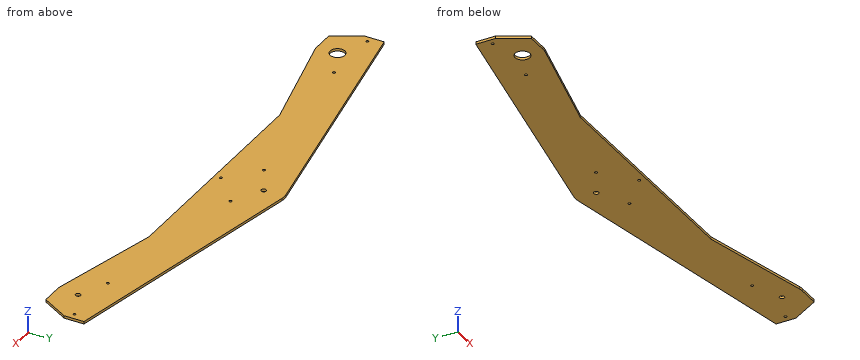
from build123d import *

# Parameters (mm, degrees)
MODEL_R             = 14.2875
MODEL_R_2           = 4.7625
MODEL_R_3           = 2.5527
BOSS_EXTRUDE1_DEPTH = 4.7752


with BuildPart() as part:
    # Model → Boss-Extrude1 (new body)
    with BuildSketch(Plane.XY):
        with BuildLine():
            Line((379.149829152, 1141.15149464), (590.378339475, 1192.375592492))
            Line((590.378339475, 1192.375592492), (814.376062419, 1192.375592492))
            Line((814.376062419, 1192.375592492), (1038.373785363, 1192.375592492))
            Line((1038.373785363, 1192.375592492), (1249.602295686, 1141.15149464))
            ThreePointArc((1249.602295686, 1141.15149464), (1254.256081724, 1140.312171612), (1258.976587117, 1140.031072925))
            Line((1258.976587117, 1140.031072925), (1298.696307446, 1140.031072925))
            Line((1298.696307446, 1140.031072925), (1328.726062419, 1192.375592492))
            Line((1328.726062419, 1192.375592492), (1328.726062419, 1230.475592492))
            Line((1328.726062419, 1230.475592492), (821.794166075, 1326.704151001))
            ThreePointArc((821.794166075, 1326.704151001), (814.376062419, 1327.401992492), (806.957958762, 1326.704151001))
            Line((806.957958762, 1326.704151001), (300.026062419, 1230.475592492))
            Line((300.026062419, 1230.475592492), (300.026062419, 1192.375592492))
            Line((300.026062419, 1192.375592492), (330.055817392, 1140.031072925))
            Line((330.055817392, 1140.031072925), (369.775537721, 1140.031072925))
            ThreePointArc((369.775537721, 1140.031072925), (374.496043114, 1140.312171612), (379.149829152, 1141.15149464))
        make_face()
        with Locations((369.877137721, 1179.807472925)):
            Circle(MODEL_R, mode=Mode.SUBTRACT)
        with Locations((814.376062419, 1287.625592492)):
            Circle(MODEL_R_2, mode=Mode.SUBTRACT)
        with Locations((1258.874987117, 1179.807472925)):
            Circle(MODEL_R_2, mode=Mode.SUBTRACT)
        with Locations((1201.72498751, 1205.075592492)):
            Circle(MODEL_R_3, mode=Mode.SUBTRACT)
        with Locations((1316.024986723, 1205.075592492)):
            Circle(MODEL_R_3, mode=Mode.SUBTRACT)
        with Locations((757.227138115, 1255.875592492)):
            Circle(MODEL_R_3, mode=Mode.SUBTRACT)
        with Locations((871.524986723, 1255.875592492)):
            Circle(MODEL_R_3, mode=Mode.SUBTRACT)
        with Locations((814.376062419, 1205.075592492)):
            Circle(MODEL_R_3, mode=Mode.SUBTRACT)
        with Locations((312.727138115, 1205.075592492)):
            Circle(MODEL_R_3, mode=Mode.SUBTRACT)
        with Locations((427.027137328, 1205.075592492)):
            Circle(MODEL_R_3, mode=Mode.SUBTRACT)
    extrude(amount=BOSS_EXTRUDE1_DEPTH)


solid = part.part
Design review of the part built by this model. Coordinates are the model's own, in mm. Give positions to 0.01 mm unless a question says otherwise; leave off trailing zeros. Loops run counter-clockwise (first coordinate to the right, second up) from the corner with the lowest first, then second, coordinate; pieces in that order, holes last. Notation, with made-up numbers: M -30.5,-38 L -4.5,-38 A10 ccw -4.5,-29 Z; hole C -18,52.25 d2. An arc over 180 degrees is marked long. Answer as a JSON object with one key per item and string values.
Item 1: We need section A-A (z = 3.8). Count the separate pieces of the cut face and the enclosed holes in it, and give its area (3 significant figures).
Output values:
{"separate pieces": "1", "enclosed holes": "10", "area": "106,000 mm2"}
Item 2: For P1, Ø6, axis at x = 603.5, y = 1260.5, coming from the -Z side; P2, Ø3, axis at x = 757.23, y = 1255.88, coming from the -Z side, all flat-tipped, find the tip position at first contact; note any pin that passes through.
Output values:
{"P1": "stops at z = 0", "P2": "passes through"}
Item 3: We need section B-B (x = 657). State the section outline as (y, z) points, and give its area (3 significant figures).
Output values:
{"outline": "M 1192.38,0 L 1298.24,0 L 1298.24,4.78 L 1192.38,4.78 Z", "area": "506 mm2"}
Item 4: Wall thickness on line 1 along X through (y, z) = (1203.5, 3.25); line 2 along Y through (x, z) = (1234, 1.35); line 3 along Y through (x, z) = (808, 1.65): over which ranges is each line inside the solid? List them lowest first.
Output values:
{"line 1": "x = 300.03 to 310.72, 314.74 to 425.02, 429.04 to 812.37, 816.38 to 1199.72, 1203.73 to 1314.02, 1318.03 to 1328.73", "line 2": "y = 1144.94 to 1248.46", "line 3": "y = 1192.38 to 1326.89"}
Item 5: We need section C-C (x = 508). State the section outline as (y, z) points.
Output values:
{"outline": "M 1172.4,0 L 1269.95,0 L 1269.95,4.78 L 1172.4,4.78 Z"}
